```python
from build123d import *

# Parameters (mm, degrees)
SKETCH1_R                = 4.5
BOSS_EXTRUDE1_DEPTH      = 10
BOSS_EXTRUDE1_DEPTH_BACK = 10
SKETCH2_R                = 4.5
SKETCH2_R_2              = 3.5
CUT_EXTRUDE1_DEPTH       = 4
CUT_EXTRUDE1_DEPTH_BACK  = 4
SKETCH3_R                = 1
CUT_EXTRUDE2_DEPTH       = 20
SKETCH4_R                = 2
CUT_EXTRUDE3_DEPTH       = 12
SKETCH5_R                = 1.25
CUT_EXTRUDE4_DEPTH       = 10
CUT_EXTRUDE4_DEPTH_BACK  = 10


with BuildPart() as part:
    # Sketch1 → Boss-Extrude1 (new body, two sides)
    with BuildSketch(Plane.XY) as boss_extrude1_sk:
        Circle(SKETCH1_R)
    extrude(amount=BOSS_EXTRUDE1_DEPTH)
    extrude(boss_extrude1_sk.sketch, amount=-BOSS_EXTRUDE1_DEPTH_BACK)

    # Sketch2 → Cut-Extrude1 (cut, two sides)
    with BuildSketch(Plane.XY) as cut_extrude1_sk:
        Circle(SKETCH2_R)
        Circle(SKETCH2_R_2, mode=Mode.SUBTRACT)
    extrude(amount=CUT_EXTRUDE1_DEPTH, mode=Mode.SUBTRACT)
    extrude(cut_extrude1_sk.sketch, amount=-CUT_EXTRUDE1_DEPTH_BACK, mode=Mode.SUBTRACT)

    # Sketch3 → Cut-Extrude2 (cut)
    with BuildSketch(Plane.XY.offset(10)):
        Circle(SKETCH3_R)
    extrude(amount=-CUT_EXTRUDE2_DEPTH, mode=Mode.SUBTRACT)

    # Sketch4 → Cut-Extrude3 (cut)
    with BuildSketch(Plane(origin=(0, 0, -10), x_dir=(-1, 0, 0), z_dir=(0, 0, -1))):
        Circle(SKETCH4_R)
    extrude(amount=-CUT_EXTRUDE3_DEPTH, mode=Mode.SUBTRACT)

    # Sketch5 → Cut-Extrude4 (cut, two sides)
    with BuildSketch(Plane(origin=(0, 0, 0), x_dir=(1, 0, 0), z_dir=(0, 1, 0))) as cut_extrude4_sk:
        with Locations((0, 7)):
            Circle(SKETCH5_R)
        with Locations((0, -7)):
            Circle(SKETCH5_R)
    extrude(amount=CUT_EXTRUDE4_DEPTH, mode=Mode.SUBTRACT)
    extrude(cut_extrude4_sk.sketch, amount=-CUT_EXTRUDE4_DEPTH_BACK, mode=Mode.SUBTRACT)


solid = part.part
```
The listing builds one solid part. Answer for the finished solid, in the listing's coordinates (mm). A direction names the side the tool comes from. Round coordinates to 2 decimals unless told otherwise and drop trailing zeros. Loops run counter-clockwise (first coordinate to the right, second up) from the corner with the lowest first, then second, coordinate; pieces in that order, holes last. Notation, with made-up numbers: (-30, 30) - (-6, 30) arc R24 ccw to (-6, 59) - close; hole circle Ø6 at (55, -22). An arc over 180 degrees is marked (long way). Return JSON: item names as keys, results as strings. Group by question number.
1. The part is cut by section D-D on y = -1.25. Determine the outline of the cut face in (x, z), then the cut area to 3 significant figures.
2. Consider probe 1 along Z at (x, y) = (0, -3.1); probe 2 along Z at (x, y) = (-3, -3.25); probe 3 along Y at (x, z) = (0, 2.95). Determine where each line is inside the solid, lowest interval first.
3. The part is cut by section C-C on x = 0. State how many separate pieces and enclosed holes the cut face has, then the cut area to 3 significant figures.
4. The part is cut by section A-A on z = -7. Determine the outline of the cut face in (x, y), then the cut area to 3 significant figures.
5. The part is cut by section B-B on y = 0.75. Determine the outline of the cut face in (x, z), then the cut area to 3 significant figures.
6. The mould has two halves that part along X. Classify faces 4 (the cylindrical face through (1.155, -3.012, -6.521)), 5 (the flat face through (2, -1, -10)), 6 (the cylindrical face through (3.233, -1.341, 0.056)): pulls with the +X half, pulls with the -X half, needs draft (parallel to the pull), parting line crosses it, or undercut.
7. Each of these flat-tipped pins is pushed along its axis until it touches: P1, Ø2, axis at x = -2.5, z = -2.5, coming from the +Y side; P2, Ø3, axis at x = 0, y = 0, coming from the -Z side; P3, Ø3, axis at x = 0, z = -7, coming from the -Y side; P4, Ø1.5, axis at y = -2.5, z = 6, coming from the -X side. Where does it stop, or does it pass through?
8. Which of the six approach directions +Z, -Z, +X, -X, +Y, -Y give full straight-line access (tool end or side, diameter ignored) to faces 1 (the flat face through (0, -4, 4)), 2 (the cylindrical face through (1, 0, 4)), 3 (the flat face through (-1, -1, 2))?
Resolved:
{
 "1": {"outline": "(-4.32, -10) - (-1.56, -10) - (-1.56, 2) - (1.56, 2) - (1.56, -10) - (4.32, -10) - (4.32, -4) - (3.27, -4) - (3.27, 4) - (4.32, 4) - (4.32, 10) - (-4.32, 10) - (-4.32, 4) - (-3.27, 4) - (-3.27, -4) - (-4.32, -4) - close; hole circle Ø2.5 at (0, 7)", "area": "114 mm²"},
 "2": {"probe 1": "z = -10 to -8.25, -5.75 to 5.75, 8.25 to 10", "probe 2": "z = -10 to -4, 4 to 10", "probe 3": "y = -3.5 to -1, 1 to 3.5"},
 "3": {"separate pieces": "6", "enclosed holes": "0", "area": "70.0 mm²"},
 "4": {"outline": "(-1.25, -4.32) - (-1.25, -1.56) arc R2 cw to (-1.25, 1.56) - (-1.25, 4.32) arc R4.5 ccw to start; (1.25, -4.32) arc R4.5 ccw to (1.25, 4.32) - (1.25, 1.56) arc R2 cw to (1.25, -1.56) - close", "area": "38.1 mm²"},
 "5": {"outline": "(-4.44, -10) - (-1.85, -10) - (-1.85, 2) - (-0.66, 2) - (-0.66, 5.94) arc R1.25 cw to (-0.66, 8.06) - (-0.66, 10) - (-4.44, 10) - (-4.44, 4) - (-3.42, 4) - (-3.42, -4) - (-4.44, -4) - close; (0.66, 2) - (1.85, 2) - (1.85, -10) - (4.44, -10) - (4.44, -4) - (3.42, -4) - (3.42, 4) - (4.44, 4) - (4.44, 10) - (0.66, 10) - (0.66, 8.06) arc R1.25 cw to (0.66, 5.94) - close", "area": "104 mm²"},
 "6": {"face 4": "undercut", "face 5": "needs draft", "face 6": "parting line crosses it"},
 "7": {"P1": "stops at y = 3.16", "P2": "stops at z = 2", "P3": "stops at y = -4.5", "P4": "stops at x = -4.15"},
 "8": {"face 1": "none", "face 2": "+Z, -Z", "face 3": "-Z"}
}
